from build123d import *

# Parameters (mm, degrees)
BOSS_EXTRUDE1_DEPTH = 25
SKETCH2_R           = 11.15
CUT_EXTRUDE1_DEPTH  = 7
CUT_EXTRUDE2_DEPTH  = 8.75
CUT_EXTRUDE3_DEPTH  = 8.75
SKETCH5_W           = 25
SKETCH5_H           = 20.5
CUT_EXTRUDE4_DEPTH  = 8
SKETCH9_R           = 2.5
CUT_EXTRUDE5_DEPTH  = 2
CUT_EXTRUDE6_REACH  = 18.25
SKETCH10_R          = 1.25
SKETCH13_R          = 2.4
CUT_EXTRUDE7_DEPTH  = 4.5
SKETCH14_R          = 1.5
CUT_EXTRUDE8_DEPTH  = 2
CUT_EXTRUDE10_DEPTH = 20
BOSS_EXTRUDE2_DEPTH = 20
SKETCH18_W          = 45
SKETCH18_H          = 15
CUT_EXTRUDE11_DEPTH = 5
BOSS_EXTRUDE3_DEPTH = 20


with BuildPart() as part:
    # Sketch1 → Boss-Extrude1 (new body)
    with BuildSketch(Plane(origin=(0, 0, 0), x_dir=(1, 0, 0), z_dir=(0, 1, 0))):
        with BuildLine():
            Line((-80, 10), (80, 10))
            ThreePointArc((80, 10), (90, 0), (80, -10))
            Line((80, -10), (-80, -10))
            ThreePointArc((-80, -10), (-90, 0), (-80, 10))
        make_face()
    extrude(amount=BOSS_EXTRUDE1_DEPTH)

    # Sketch2 → Cut-Extrude1 (cut)
    with BuildSketch(Plane.XY.offset(10)):
        with Locations((0, 12.5)):
            Circle(SKETCH2_R)
    extrude(amount=-CUT_EXTRUDE1_DEPTH, mode=Mode.SUBTRACT)

    # Sketch3 → Cut-Extrude2 (cut)
    with BuildSketch(Plane(origin=(0, 25, 0), x_dir=(1, 0, 0), z_dir=(0, 1, 0))):
        with BuildLine():
            Line((-20, 10), (-20, -10))
            Line((-20, -10), (-80, -10))
            ThreePointArc((-80, -10), (-90, 0), (-80, 10))
            Line((-80, 10), (-20, 10))
        make_face()
        with BuildLine():
            Line((20, 10), (20, -10))
            Line((20, -10), (80, -10))
            ThreePointArc((80, -10), (90, 0), (80, 10))
            Line((80, 10), (20, 10))
        make_face()
    extrude(amount=-CUT_EXTRUDE2_DEPTH, mode=Mode.SUBTRACT)

    # Sketch4 → Cut-Extrude3 (cut)
    with BuildSketch(Plane.XZ):
        with BuildLine():
            Line((20, 10), (20, -10))
            Line((20, -10), (80, -10))
            ThreePointArc((80, -10), (90, 0), (80, 10))
            Line((80, 10), (20, 10))
        make_face()
        with BuildLine():
            Line((-20, 10), (-20, -10))
            Line((-20, -10), (-80, -10))
            ThreePointArc((-80, -10), (-90, 0), (-80, 10))
            Line((-80, 10), (-20, 10))
        make_face()
    extrude(amount=-CUT_EXTRUDE3_DEPTH, mode=Mode.SUBTRACT)

    # Sketch5 → Cut-Extrude4 (cut)
    with BuildSketch(Plane(origin=(0, 0, -10), x_dir=(-1, 0, 0), z_dir=(0, 0, -1))):
        with Locations((0, 12.5)):
            Rectangle(SKETCH5_W, SKETCH5_H)
    extrude(amount=-CUT_EXTRUDE4_DEPTH, mode=Mode.SUBTRACT)

    # Sketch9 → Cut-Extrude5 (cut)
    with BuildSketch(Plane(origin=(0, 16.25, 0), x_dir=(1, 0, 0), z_dir=(0, 1, 0))):
        with Locations((-80, 0)):
            Circle(SKETCH9_R)
        with Locations((80, 0)):
            Circle(SKETCH9_R)
    extrude(amount=-CUT_EXTRUDE5_DEPTH, mode=Mode.SUBTRACT)

    # Sketch10 → Cut-Extrude6 (cut, up to next)
    with BuildSketch(Plane(origin=(0, 16.25, 0), x_dir=(1, 0, 0), z_dir=(0, 1, 0)), mode=Mode.PRIVATE) as cut_extrude6_sk1:
        with Locations((-75.56, 4.44)):
            Circle(SKETCH10_R)
    cut_extrude6_tool1 = extrude(cut_extrude6_sk1.sketch, amount=-CUT_EXTRUDE6_REACH, mode=Mode.PRIVATE) & part.part
    add(cut_extrude6_tool1.solids().sort_by_distance((-75.56, 16.25, -4.44))[0], mode=Mode.SUBTRACT)
    # Sketch10 → Cut-Extrude6 (cut, up to next)
    with BuildSketch(Plane(origin=(0, 16.25, 0), x_dir=(1, 0, 0), z_dir=(0, 1, 0)), mode=Mode.PRIVATE) as cut_extrude6_sk2:
        with Locations((-75.56, -4.44)):
            Circle(SKETCH10_R)
    cut_extrude6_tool2 = extrude(cut_extrude6_sk2.sketch, amount=-CUT_EXTRUDE6_REACH, mode=Mode.PRIVATE) & part.part
    add(cut_extrude6_tool2.solids().sort_by_distance((-75.56, 16.25, 4.44))[0], mode=Mode.SUBTRACT)
    # Sketch10 → Cut-Extrude6 (cut, up to next)
    with BuildSketch(Plane(origin=(0, 16.25, 0), x_dir=(1, 0, 0), z_dir=(0, 1, 0)), mode=Mode.PRIVATE) as cut_extrude6_sk3:
        with Locations((-84.44, -4.44)):
            Circle(SKETCH10_R)
    cut_extrude6_tool3 = extrude(cut_extrude6_sk3.sketch, amount=-CUT_EXTRUDE6_REACH, mode=Mode.PRIVATE) & part.part
    add(cut_extrude6_tool3.solids().sort_by_distance((-84.44, 16.25, 4.44))[0], mode=Mode.SUBTRACT)
    # Sketch10 → Cut-Extrude6 (cut, up to next)
    with BuildSketch(Plane(origin=(0, 16.25, 0), x_dir=(1, 0, 0), z_dir=(0, 1, 0)), mode=Mode.PRIVATE) as cut_extrude6_sk4:
        with Locations((-84.44, 4.44)):
            Circle(SKETCH10_R)
    cut_extrude6_tool4 = extrude(cut_extrude6_sk4.sketch, amount=-CUT_EXTRUDE6_REACH, mode=Mode.PRIVATE) & part.part
    add(cut_extrude6_tool4.solids().sort_by_distance((-84.44, 16.25, -4.44))[0], mode=Mode.SUBTRACT)
    # Sketch10 → Cut-Extrude6 (cut, up to next)
    with BuildSketch(Plane(origin=(0, 16.25, 0), x_dir=(1, 0, 0), z_dir=(0, 1, 0)), mode=Mode.PRIVATE) as cut_extrude6_sk5:
        with Locations((84.44, 4.44)):
            Circle(SKETCH10_R)
    cut_extrude6_tool5 = extrude(cut_extrude6_sk5.sketch, amount=-CUT_EXTRUDE6_REACH, mode=Mode.PRIVATE) & part.part
    add(cut_extrude6_tool5.solids().sort_by_distance((84.44, 16.25, -4.44))[0], mode=Mode.SUBTRACT)
    # Sketch10 → Cut-Extrude6 (cut, up to next)
    with BuildSketch(Plane(origin=(0, 16.25, 0), x_dir=(1, 0, 0), z_dir=(0, 1, 0)), mode=Mode.PRIVATE) as cut_extrude6_sk6:
        with Locations((84.44, -4.44)):
            Circle(SKETCH10_R)
    cut_extrude6_tool6 = extrude(cut_extrude6_sk6.sketch, amount=-CUT_EXTRUDE6_REACH, mode=Mode.PRIVATE) & part.part
    add(cut_extrude6_tool6.solids().sort_by_distance((84.44, 16.25, 4.44))[0], mode=Mode.SUBTRACT)
    # Sketch10 → Cut-Extrude6 (cut, up to next)
    with BuildSketch(Plane(origin=(0, 16.25, 0), x_dir=(1, 0, 0), z_dir=(0, 1, 0)), mode=Mode.PRIVATE) as cut_extrude6_sk7:
        with Locations((75.56, -4.44)):
            Circle(SKETCH10_R)
    cut_extrude6_tool7 = extrude(cut_extrude6_sk7.sketch, amount=-CUT_EXTRUDE6_REACH, mode=Mode.PRIVATE) & part.part
    add(cut_extrude6_tool7.solids().sort_by_distance((75.56, 16.25, 4.44))[0], mode=Mode.SUBTRACT)
    # Sketch10 → Cut-Extrude6 (cut, up to next)
    with BuildSketch(Plane(origin=(0, 16.25, 0), x_dir=(1, 0, 0), z_dir=(0, 1, 0)), mode=Mode.PRIVATE) as cut_extrude6_sk8:
        with Locations((75.56, 4.44)):
            Circle(SKETCH10_R)
    cut_extrude6_tool8 = extrude(cut_extrude6_sk8.sketch, amount=-CUT_EXTRUDE6_REACH, mode=Mode.PRIVATE) & part.part
    add(cut_extrude6_tool8.solids().sort_by_distance((75.56, 16.25, -4.44))[0], mode=Mode.SUBTRACT)

    # Sketch13 → Cut-Extrude7 (cut)
    with BuildSketch(Plane.XZ.offset(-8.75)):
        with Locations((-75.56, 4.44)):
            Circle(SKETCH13_R)
        with Locations((-75.56, -4.44)):
            Circle(SKETCH13_R)
        with Locations((-84.44, -4.44)):
            Circle(SKETCH13_R)
        with Locations((-84.44, 4.44)):
            Circle(SKETCH13_R)
        with Locations((84.44, 4.44)):
            Circle(SKETCH13_R)
        with Locations((84.44, -4.44)):
            Circle(SKETCH13_R)
        with Locations((75.56, -4.44)):
            Circle(SKETCH13_R)
        with Locations((75.56, 4.44)):
            Circle(SKETCH13_R)
    extrude(amount=-CUT_EXTRUDE7_DEPTH, mode=Mode.SUBTRACT)

    # Sketch14 → Cut-Extrude8 (cut)
    with BuildSketch(Plane(origin=(0, 25, 0), x_dir=(1, 0, 0), z_dir=(0, 1, 0))):
        with Locations((-8.25, 7.46)):
            Circle(SKETCH14_R)
        with Locations((8.25, 7.46)):
            Circle(SKETCH14_R)
    extrude(amount=-CUT_EXTRUDE8_DEPTH, mode=Mode.SUBTRACT)

    # Sketch16 → Cut-Extrude10 (cut)
    with BuildSketch(Plane(origin=(0, 0, -10), x_dir=(-1, 0, 0), z_dir=(0, 0, -1))):
        with BuildLine():
            Line((-12.5, 25), (-20, 25))
            Line((-20, 25), (-20, 16.25))
            add(Edge.make_bspline(
                [(-20, 16.25), (-20, 20.091476857), (-17.882145689, 25), (-12.5, 25)],
                knots=[0, 0, 0, 0, 1, 1, 1, 1], degree=3))
        make_face()
        with BuildLine():
            Line((12.5, 25), (20, 25))
            Line((20, 25), (20, 16.25))
            add(Edge.make_bspline(
                [(20, 16.25), (20, 20.091476857), (17.882145689, 25), (12.5, 25)],
                knots=[0, 0, 0, 0, 1, 1, 1, 1], degree=3))
        make_face()
        with BuildLine():
            Line((20, 0), (20, 8.75))
            add(Edge.make_bspline(
                [(20, 8.75), (20, 4.908523143), (17.882145689, 0), (12.5, 0)],
                knots=[0, 0, 0, 0, 1, 1, 1, 1], degree=3))
            Line((12.5, 0), (20, 0))
        make_face()
        with BuildLine():
            Line((-20, 0), (-20, 8.75))
            add(Edge.make_bspline(
                [(-20, 8.75), (-20, 4.908523143), (-17.882145689, 0), (-12.5, 0)],
                knots=[0, 0, 0, 0, 1, 1, 1, 1], degree=3))
            Line((-12.5, 0), (-20, 0))
        make_face()
    extrude(amount=-CUT_EXTRUDE10_DEPTH, mode=Mode.SUBTRACT)

    # Sketch17 → Boss-Extrude2 (add)
    with BuildSketch(Plane(origin=(0, 0, -10), x_dir=(-1, 0, 0), z_dir=(0, 0, -1))):
        Polygon((12.5, 0), (12.5, -5), (7.5, -5), (7.5, -3.25), (10, -3.25), (10, -0.75), (-10, -0.75), (-10, -3.25), (-7.5, -3.25), (-7.5, -5), (-12.5, -5), (-12.5, 0), align=None)
    extrude(amount=-BOSS_EXTRUDE2_DEPTH)

    # Sketch18 → Cut-Extrude11 (cut)
    with BuildSketch(Plane(origin=(0, 16.25, 0), x_dir=(1, 0, 0), z_dir=(0, 1, 0))):
        with Locations((47.5, 0)):
            Rectangle(SKETCH18_W, SKETCH18_H)
        with Locations((-47.5, 0)):
            Rectangle(SKETCH18_W, SKETCH18_H)
    extrude(amount=-CUT_EXTRUDE11_DEPTH, mode=Mode.SUBTRACT)

    # Sketch20 → Boss-Extrude3 (add)
    with BuildSketch(Plane.XY.offset(10)):
        Polygon((-25, 11.25), (-25, 16.25), (-35.722534603, 11.25), align=None)
        Polygon((-70, 11.25), (-59.277465397, 11.25), (-70, 16.25), align=None)
        Polygon((25, 11.25), (35.722534603, 11.25), (25, 16.25), align=None)
        Polygon((70, 11.25), (70, 16.25), (59.277465397, 11.25), align=None)
    extrude(amount=-BOSS_EXTRUDE3_DEPTH)


solid = part.part
Part model, mm, in its own coordinate system. A direction names the side the tool comes from. Give positions to 0.01 mm unless a question says otherwise; leave off trailing zeros. Loops run counter-clockwise (first coordinate to the right, second up) from the corner with the lowest first, then second, coordinate; pieces in that order, holes last. Notation, with made-up numbers: M -34.5,22.5 L 7.5,22.5 A20 cw 7.5,40.5 Z; hole C 23,17 d1. An arc over 180 degrees is marked long. Put each result on its own line as item: value. Start each with the question number.
1) Pull direction Y, two halves, no side cores. Call faces 6 (the flat face through (-8, 23, -7)), 7 (the cylindrical face through (-90, 12, 0)), 8 (the cylindrical face through (10.635, 15.849, 6.549)), 9 (the flat face through (0, 2.25, -6)): +Y half, -Y half, draft (parallel to the pull), parting line (faces both ways), or undercut.
2) Flat gauge pins, fed straight in: pin 1 (4.5 mm diameter, centred on x = -84.44, z = 4.44, fed in from +Y); pin 2 (5.5 mm diameter, centred on x = 75.56, z = -4.44, fed in from -Y); pin 3 (1.5 mm diameter, centred on x = 8.5, z = -7.5, fed in from +Y). Where does each tip first touch, or does it go through?
3) Probe probe 1 along Z at (x, y) = (-75.56, 14.65); probe 2 along X at (y, z) = (-3, 4.75); probe 3 along Z at (x, y) = (-61, 16). List the from-to ranges inside material, lowest first.
4) 3-axis set-ups, long thin cutter, end or side, ignore diameter. For faces 1 (the cylindrical face through (77.5, 15.3, -0.1)), 2 (the flat face through (55, 8.75, 0)), 3 (the flat face through (55, 16.25, 9)), 4 (the flat face through (-55, 16.25, 9)), 5 (the cylindrical face through (73.162, 10.968, 4.546)): which of +Z, -Z, +X, -X, +Y, -Y reach the whole face in a straight line?
5) Saw through at B-B (x = 0). List the corners of the cut face in (y, z).
6) Saw through at A-A (x = -48.5). List the corners of the cut face in (y, z), then the cut area to 3 significant figures.
Numbers:
1. face 6: +Y half
1. face 7: draft
1. face 8: undercut
1. face 9: undercut
2. pin 1: y = 16.25
2. pin 2: y = 8.75
2. pin 3: y = 23
3. probe 1: -10 to -5.69, -3.19 to 3.19, 5.69 to 10
3. probe 2: -12.5 to -10, 10 to 12.5
3. probe 3: -10 to -7.5, 7.5 to 10
4. face 1: +Y
4. face 2: +Z, -Z, +X, -Y
4. face 3: +Z, -Z, +X, +Y
4. face 4: +Z, -Z, -X, +Y
4. face 5: -Y
5. outline: M -0.75,-10 L 2.25,-10 L 2.25,-2 L 22.75,-2 L 22.75,-10 L 25,-10 L 25,10 L 23.65,10 L 23.65,3 L 1.35,3 L 1.35,10 L -0.75,10 Z
6. outline: M 8.75,-10 L 16.25,-10 L 16.25,-7.5 L 11.25,-7.5 L 11.25,7.5 L 16.25,7.5 L 16.25,10 L 8.75,10 Z
6. area: 75.0 mm^2
